from build123d import *

# Parameters (mm, degrees)
F0_W        = 152.4
F0_H        = 152.4
F1_DEPTH    = 6.35
F2_W        = 152.4
F2_H        = 6.35
F3_DEPTH    = 241.3
F5_T1_DEPTH = 404.9366591478
F6_W        = 6.35
F6_H        = 115.4995709658
F7_DEPTH    = 25.4
F8_R        = 5.08
F9_DEPTH    = 6.35
F11_DEPTH   = 6.35


# Not quite as in the source:
# - a fillet or chamfer that OpenCascade refuses, or shapes differently, is made with other operations: its cross-section is extruded or revolved along the edge and cut away or added


with BuildPart() as f1:
    # F0 (on Top) → F1 (new body)
    with BuildSketch(Plane.XY):
        with Locations((2.7477228088, -4.3853670359)):
            Rectangle(F0_W, F0_H)
    extrude(amount=F1_DEPTH)

    # F2 (on face) → F3 (join)
    with BuildSketch(Plane.XY.offset(6.35)):
        with Locations((2.7477228088, -77.4103670359)):
            Rectangle(F2_W, F2_H)
    extrude(amount=F3_DEPTH)

    # F5: fillet of radius 79.7173318296 on 2 edges, made by hand

    # F5_s2 → F5_t1 (cut)
    with BuildSketch(Plane.XZ.offset(-125.057962538)):
        with BuildLine():
            ThreePointArc((-73.4522771912, 167.9326681704), (-50.1036112765, 224.3013340852), (6.2650546383, 247.65))
            Line((6.2650546383, 247.65), (-73.4522771912, 247.65))
            Line((-73.4522771912, 247.65), (-73.4522771912, 167.9326681704))
        make_face()
        with BuildLine():
            ThreePointArc((78.9477228088, 167.9326681704), (55.599056894, 224.3013340852), (-0.7696090208, 247.65))
            Line((-0.7696090208, 247.65), (78.9477228088, 247.65))
            Line((78.9477228088, 247.65), (78.9477228088, 167.9326681704))
        make_face()
    extrude(amount=F5_T1_DEPTH, mode=Mode.SUBTRACT)

    # F6 (on face) → F7 (cut)
    with BuildSketch(Plane.XZ.offset(80.5853670359)):
        with Locations((2.7477228088, 153.0246064067)):
            Rectangle(F6_W, F6_H)
    extrude(amount=-F7_DEPTH, mode=Mode.SUBTRACT)

    # F8
    f8_edges = [f1.edges().sort_by_distance(p)[0] for p in [
        (78.947723, 71.814633, 3.175),
        (-73.452277, 71.814633, 3.175),
    ]]
    fillet(f8_edges, radius=F8_R)

    # F4 (on face) → F9 (join)
    with BuildSketch(Plane.YZ.offset(78.9477228088)):
        Polygon((-74.2353670359, 6.35), (0, 6.35), (-74.2353670359, 38.8328842819), align=None)
    extrude(amount=-F9_DEPTH)

    # F10 (on face) → F11 (join)
    with BuildSketch(Plane(origin=(-73.4522771912, 0, 0), x_dir=(0, -1, 0), z_dir=(-1, 0, 0))):
        Polygon((74.2353670359, 6.35), (74.2353670359, 38.6480651796), (0, 6.35), align=None)
    extrude(amount=-F11_DEPTH)


solid = f1.part
Build history of the part. All positions in model axes, mm. A direction names the side the tool comes from. Coordinates: 2 decimals unless noted, no trailing zeros. Order: outer loops, then holes, each group sorted by start corner. A loop starts at its lowest first (then second) coordinate and runs counter-clockwise, first axis right, second up. Notation, with made-up numbers: (-20.5, -3.5) -> (21.5, -3.5) arc R25 ccw to (21.5, 27.5) -> close; hole circle Ø5 at (-3.75, 1.25). An arc over 180 degrees is marked (long way). One line per item, written item: value.
(1) Slice it at B-B, the plane y = -67.5. List the corners of the cut face in (x, z), plus the area to 3 significant figures.
Checked values:
outline: (-73.45, 0) -> (78.95, 0) -> (78.95, 35.89) -> (72.6, 35.89) -> (72.6, 6.35) -> (-67.1, 6.35) -> (-67.1, 35.72) -> (-73.45, 35.72) -> close
area: 1,340 mm2
(2) Tool access for faces 4 (the flat face through (19, -74.235, 125)), 5 (the flat face through (3, -77, 210.774)), 6 (the flat face through (-73.452, -45, 22)): list every direction of +Z, -Z, +X, -X, +Y, -Y with a clear straight run to the whole face (end or side of a thin tool).
Checked values:
face 4: +Z, +Y
face 5: +Y, -Y
face 6: +Z, -Z, -X, +Y, -Y
(3) Mould opens along X. For faces 1 (the cylindrical face through (-51.919, -77.366, 222.425)), 2 (the flat face through (2, -80.585, 95)), 3 (the flat face through (2, 0, 6.35)) say: pulls with the +X half, pulls with the -X half, needs draft (parallel to the pull), parting line crosses it, or undercut.
Checked values:
face 1: pulls with the -X half
face 2: needs draft
face 3: undercut
(4) Drop flat-ended pins along their axis: pin 1 Ø4 at (x, z) = (60.5, 205) entering from +Y; pin 2 Ø2 at (x, y) = (43, 32.5) entering from +Z. Give the stop position or say it passes through.
Checked values:
pin 1: y = -74.24
pin 2: z = 6.35
(5) Slice it at C-C, the plane z = 51. List the corners of the cut face in (x, y).
Checked values:
outline: (-73.45, -80.59) -> (78.95, -80.59) -> (78.95, -74.24) -> (-73.45, -74.24) -> close
(6) Slice it at A-A, the plane z = 129. List the corners of the cut face in (x, y), plus the area to 3 significant figures.
Checked values:
outline: (-73.45, -80.59) -> (-0.43, -80.59) -> (-0.43, -74.24) -> (-73.45, -74.24) -> close; (5.92, -80.59) -> (78.95, -80.59) -> (78.95, -74.24) -> (5.92, -74.24) -> close
area: 927 mm2
(7) Probe line 1 (Z direction, x = 33, y = -34.5); line 2 (Y direction, x = -5.5, z = 148). List the from-to ranges inside material, lowest first. Write a range as [from, to].
Checked values:
line 1: [0, 6.35]
line 2: [-80.59, -74.24]
(8) Slice it at D-D, the plane x = -60.5. List the corners of the cut face in (y, z), plus the area to 3 significant figures.
Checked values:
outline: (-80.59, 0) -> (71.81, 0) -> (71.81, 6.35) -> (-74.24, 6.35) -> (-74.24, 211.49) -> (-80.59, 211.49) -> close
area: 2,270 mm2
